Check sheet for the modelled part. Datum: model origin and axes. Units: mm. Face numbers are marked on the shaded views. Coordinates: 2 decimals unless noted, no trailing zeros. Loops run counter-clockwise (first coordinate to the right, second up) from the corner with the lowest first, then second, coordinate; pieces in that order, holes last. Notation, with made-up numbers: (11.5, -30.75) -> (63.5, -30.75) arc R36 cw to (63.5, 8.25) -> close; hole circle Ø4 at (-18.75, 70.25). An arc over 180 degrees is marked (long way). Use one line per item in the form item = value.
from build123d import *

# Parameters (mm, degrees)
F0_W     = 752.983
F0_H     = 151.4094
F0_W_2   = 112.649
F0_H_2   = 69.1896
F1_DEPTH = 0.7239
F2_DEPTH = 10.16
F3_DEPTH = 10.16
F4_DEPTH = 10.16
F5_DEPTH = 10.16
F6_R     = 1.905
F7_DEPTH = 0.7249
F8_R     = 5.08


with BuildPart() as f1:
    # F0 (on Front) → F1 (new body)
    with BuildSketch(Plane.XZ):
        Rectangle(F0_W, F0_H)
        with Locations((-1.8796, 1.9177)):
            Rectangle(F0_W_2, F0_H_2, mode=Mode.SUBTRACT)
    extrude(amount=F1_DEPTH)

    # F2 (add): a face of the model
    f2_faces = [f1.faces().sort_by_distance(p)[0] for p in [
        (0, -0.36195, 75.7047),
    ]]
    extrude(f2_faces, amount=F2_DEPTH)

    # F3 (add): a face of the model
    f3_faces = [f1.faces().sort_by_distance(p)[0] for p in [
        (0, -0.36195, -75.7047),
    ]]
    extrude(f3_faces, amount=F3_DEPTH)

    # F4 (add): a face of the model
    f4_faces = [f1.faces().sort_by_distance(p)[0] for p in [
        (376.4915, -0.36195, 0),
    ]]
    extrude(f4_faces, amount=F4_DEPTH)

    # F5 (add): a face of the model
    f5_faces = [f1.faces().sort_by_distance(p)[0] for p in [
        (-376.4915, -0.36195, 0),
    ]]
    extrude(f5_faces, amount=F5_DEPTH)

    # F6 (on face) → F7 (cut, through all)
    with BuildSketch(Plane(origin=(0, 0, 0), x_dir=(-1, 0, 0), z_dir=(0, 1, 0))):
        with Locations((-381.5715, 80.7847)):
            Circle(F6_R)
        with Locations((1.8796, 80.7847)):
            Circle(F6_R)
        with Locations((381.5715, 80.7847)):
            Circle(F6_R)
        with Locations((-381.5715, -80.7847)):
            Circle(F6_R)
        with Locations((1.8796, -80.7847)):
            Circle(F6_R)
        with Locations((381.5715, -80.7847)):
            Circle(F6_R)
        with Locations((154.2796, 80.7847)):
            Circle(F6_R)
        with Locations((229.1715, 80.7847)):
            Circle(F6_R)
        with Locations((-150.5204, 80.7847)):
            Circle(F6_R)
        with Locations((-229.1715, 80.7847)):
            Circle(F6_R)
        with Locations((-381.5715, 0)):
            Circle(F6_R)
        with Locations((381.5715, 0)):
            Circle(F6_R)
        with Locations((-229.1715, -80.7847)):
            Circle(F6_R)
        with Locations((-150.5204, -80.7847)):
            Circle(F6_R)
        with Locations((154.2796, -80.7847)):
            Circle(F6_R)
        with Locations((229.1715, -80.7847)):
            Circle(F6_R)
    extrude(amount=-F7_DEPTH, mode=Mode.SUBTRACT)

    # F8
    f8_edges = [f1.edges().sort_by_distance(p)[0] for p in [
        (386.6515, -0.36195, 85.8647),
        (386.6515, -0.36195, -85.8647),
        (-386.6515, -0.36195, -85.8647),
        (-386.6515, -0.36195, 85.8647),
    ]]
    fillet(f8_edges, radius=F8_R)


solid = f1.part
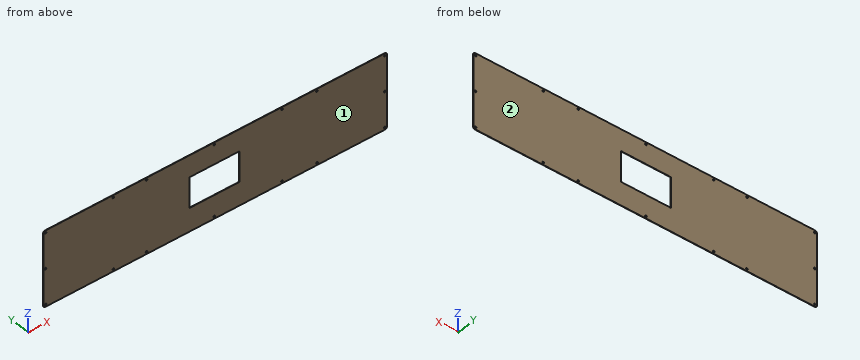
(1) Mould release check, pull along Y, two halves, no side actions. Record for the marked faces 1 and 2: +Y half, -Y half, draft (parallel to the pull), parting line (faces both ways), or undercut.
Established:
face_1 = -Y half
face_2 = +Y half
(2) Go/stop test with a flat-tipped pin: P1, Ø2.5, axis at x = -1.88, z = 80.78, coming from the -Y side. Record where the tip stops, or that it passes through.
Established:
P1 = through
(3) Scan lines: line 1 along X through (y, z) = (-0.5, -6); line 2 along Z through (x, y) = (4, -0.05). Record each from-to range of solid material in increasing order.
Established:
line_1 = -386.65 to -58.2, 54.44 to 386.65
line_2 = -85.86 to -32.68, 36.51 to 85.86
(4) Section check B-B, the plane z = 15. Record the boundary of the cut face in (x, y).
Established:
outline = (-386.65, -0.72) -> (-58.2, -0.72) -> (-58.2, 0) -> (-386.65, 0) -> close; (54.44, -0.72) -> (386.65, -0.72) -> (386.65, 0) -> (54.44, 0) -> close
(5) Section check A-A, the plane y = -0.5. Give the number of separate pieces and of enclosed holes in the cut face, plus the area to 3 significant figures.
Established:
separate_pieces = 1
enclosed_holes = 17
area = 125,000 mm²
